Could you check a few things on this model? Use its own coordinates, in mm. Face numbers are marked on the shaded views. A direction names the side the tool comes from. Coordinates: 2 decimals unless noted, no trailing zeros. Loops run counter-clockwise (first coordinate to the right, second up) from the corner with the lowest first, then second, coordinate; pieces in that order, holes last.
1) If I drill on line 1 along Y through (x, z) = (0, 8.55); line 2 along X through (y, z) = (0.5, 17); line 3 along X through (y, z) = (14.25, 17.75), over which ranges is the centre line in solid material (lowest first)?
2) Imagine slicing it at D-D on y = 5.5. Please give me the cut outline in (x, z).
3) Imagine slicing it at A-A on z = 12. Please give me the cut outline in (x, y).
4) Thinking about a two-plate mould opening in Z: for the marked faces 4, 5 and 6, which applies, released by +Z, released by -Z, zero draft, split by the parting line, or undercut?
5) Imagine slicing it at B-B on z = 5.5. Please give me the cut outline in (x, y), plus the area to 3 significant figures.
6) For the marked faces 1, 2 and 3, which set-ups out of +Z, -Z, +X, -X, +Y, -Y let a thin tool reach every point of the face, with its end or its side?
7) Will these pins go through, and if not, where does the flat tip stop? P1, Ø10.5, axis at x = -16, z = 5.5, coming from the -Y side; P2, Ø8, axis at x = 0, y = 0, coming from the +Z side; P3, Ø10, axis at y = 1, z = 13.5, coming from the -X side; P4, Ø1.5, axis at y = -6.5, z = 16, coming from the +X side.
8) Imagine slicing it at C-C on y = 0.5. Please give me the cut outline in (x, z), plus the area to 3 significant figures.
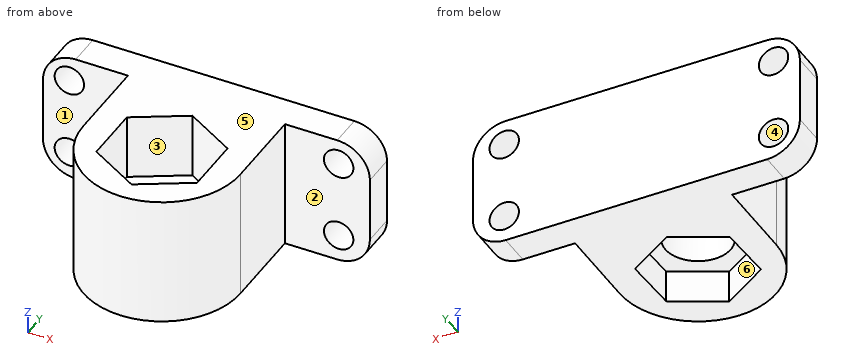
```python
from build123d import *

# Parameters (mm, degrees)
F0_R      = 5
F1_DEPTH  = 20
F2_W      = 50
F2_H      = 5
F3_DEPTH  = 20
F4_R      = 2.25
F5_DEPTH  = 25
F6_R      = 5
F8_DEPTH  = 10
F10_DEPTH = 5


with BuildPart() as f1:
    # F0 (on Top) → F1 (new body)
    with BuildSketch(Plane.XY):
        with BuildLine():
            Line((12, 18), (-12, 18))
            Line((-12, 18), (-12, 0))
            ThreePointArc((-12, 0), (0, -12), (12, 0))
            Line((12, 0), (12, 18))
        make_face()
        Circle(F0_R, mode=Mode.SUBTRACT)
    extrude(amount=F1_DEPTH)

    # F2 (on face) → F3 (join, through all)
    with BuildSketch(Plane.XY.offset(20)):
        with Locations((0, 15.5)):
            Rectangle(F2_W, F2_H)
    extrude(amount=-F3_DEPTH)

    # F4 (on face) → F5 (cut)
    with BuildSketch(Plane.XZ.offset(-13)):
        with Locations((-20.970641, 16.129617)):
            Circle(F4_R)
        with Locations((20.224099, 16.129617)):
            Circle(F4_R)
        with Locations((-20.970641, 4.11036)):
            Circle(F4_R)
        with Locations((20.224099, 4.11036)):
            Circle(F4_R)
    extrude(amount=-F5_DEPTH, mode=Mode.SUBTRACT)

    # F6
    f6_edges = [f1.edges().sort_by_distance(p)[0] for p in [
        (25, 15.5, 0),
        (-25, 15.5, 0),
        (-25, 15.5, 20),
        (25, 15.5, 20),
    ]]
    fillet(f6_edges, radius=F6_R)

    # F7 (on face) → F8 (cut)
    with BuildSketch(Plane.XY.offset(20)):
        Polygon((7.702981, 4.447318), (0, 8.894636), (-7.702981, 4.447318), (-7.702981, -4.447318), (0, -8.894636), (7.702981, -4.447318), align=None)
    extrude(amount=-F8_DEPTH, mode=Mode.SUBTRACT)

    # F9 (on face) → F10 (cut)
    with BuildSketch(Plane(origin=(0, 0, 0), x_dir=(1, 0, 0), z_dir=(0, 0, -1))):
        Polygon((-0.291229, 8.527634), (-7.530763, 4.011605), (-7.239533, -4.516029), (0.291229, -8.527634), (7.530763, -4.011605), (7.239533, 4.516029), align=None)
    extrude(amount=-F10_DEPTH, mode=Mode.SUBTRACT)


solid = f1.part
```
Filled in:
1. line 1: y = -12 to -5, 5 to 18
1. line 2: x = -12 to -7.7, 7.7 to 12
1. line 3: x = -24.18 to -22.53, -19.41 to 18.66, 21.79 to 24.18
2. outline: (-12, 0) - (-5.39, 0) - (-5.39, 5) - (5.14, 5) - (5.14, 0) - (12, 0) - (12, 20) - (5.88, 20) - (5.88, 10) - (-5.88, 10) - (-5.88, 20) - (-12, 20) - close
3. outline: (-25, 13) - (-12, 13) - (-12, 0) arc R12 ccw to (12, 0) - (12, 13) - (25, 13) - (25, 18) - (-25, 18) - close; hole (-7.7, -4.45) - (0, -8.89) - (7.7, -4.45) - (7.7, 4.45) - (0, 8.89) - (-7.7, 4.45) - close
4. face 4: undercut
4. face 5: released by +Z
4. face 6: zero draft
5. outline: (-25, 13) - (-22.74, 13) - (-22.74, 18) - (-25, 18) - close; (-19.2, 13) - (-12, 13) - (-12, 0) arc R12 ccw to (12, 0) - (12, 13) - (18.45, 13) - (18.45, 18) - (-19.2, 18) - close; (21.99, 13) - (25, 13) - (25, 18) - (21.99, 18) - close; hole circle Ø10 at (0, 0)
5. area: 674 mm2
6. face 1: +Z, -Z, -X, -Y
6. face 2: +Z, -Z, +X, -Y
6. face 3: +Z
7. P1: stops at y = -5.33
7. P2: passes through
7. P3: stops at x = -12
7. P4: stops at x = 10.53
8. outline: (-12, 0) - (-7.38, 0) - (-7.38, 5) - (-4.97, 5) - (-4.97, 10) - (-7.7, 10) - (-7.7, 20) - (-12, 20) - close; (4.97, 5) - (7.41, 5) - (7.41, 0) - (12, 0) - (12, 20) - (7.7, 20) - (7.7, 10) - (4.97, 10) - close
8. area: 202 mm2
